Build history of the part. All positions in model axes, mm. A direction names the side the tool comes from. Round coordinates to 2 decimals unless told otherwise and drop trailing zeros. Order: outer loops, then holes, each group sorted by start corner. A loop starts at its lowest first (then second) coordinate and runs counter-clockwise, first axis right, second up. Notation, with made-up numbers: (61.5, 8) -> (113.5, 8) arc R23 ccw to (113.5, 28) -> close; hole circle Ø10 at (89.5, 67.5). An arc over 180 degrees is marked (long way). Answer as a JSON object with one key per item and string values.
from build123d import *

# Parameters (mm, degrees)
SKETCH_1_R          = 1.6
EXTRUDE_1_DEPTH     = 2
CUT_EXTRUDE_1_DEPTH = 88.4814266


with BuildPart() as part:
    # 草图1 → 凸台-拉伸1 (new body)
    with BuildSketch(Plane.XY):
        Polygon((0, 0), (0, 30), (25, 68), (55, 68), (55, 58), (44.157894737, 58), (6, 0), align=None)
        with Locations((3, 25)):
            Circle(SKETCH_1_R, mode=Mode.SUBTRACT)
        with Locations((3, 5)):
            Circle(SKETCH_1_R, mode=Mode.SUBTRACT)
        with Locations((30, 65)):
            Circle(SKETCH_1_R, mode=Mode.SUBTRACT)
        with Locations((50, 65)):
            Circle(SKETCH_1_R, mode=Mode.SUBTRACT)
    extrude(amount=EXTRUDE_1_DEPTH)

    # 草图2 → 切除-拉伸1 (cut, through all)
    with BuildSketch(Plane.XY.offset(2)):
        with BuildLine():
            Line((35.120951799, 58), (38.711972457, 58))
            ThreePointArc((38.711972457, 58), (39.592204387, 57.474543727), (39.547389539, 56.450383499))
            Line((39.547389539, 56.450383499), (29.621611135, 41.363200325))
            ThreePointArc((29.621611135, 41.363200325), (28.988285582, 40.933450188), (28.236577552, 41.077399744))
            Line((28.236577552, 41.077399744), (25.730326305, 42.726249249))
            ThreePointArc((25.730326305, 42.726249249), (25.300576167, 43.359574802), (25.444525724, 44.111282833))
            Line((25.444525724, 44.111282833), (34.285534717, 57.549616501))
            ThreePointArc((34.285534717, 57.549616501), (34.646408072, 57.88023193), (35.120951799, 58))
        make_face()
        with BuildLine():
            Line((8, 11.837801866), (8, 17.296153265))
            ThreePointArc((8, 17.296153265), (8.042028946, 17.583018145), (8.164582918, 17.845769767))
            Line((8.164582918, 17.845769767), (21.597210214, 38.263363257))
            ThreePointArc((21.597210214, 38.263363257), (22.230535767, 38.693113395), (22.982243798, 38.549163838))
            Line((22.982243798, 38.549163838), (25.488495044, 36.900314333))
            ThreePointArc((25.488495044, 36.900314333), (25.918245182, 36.26698878), (25.774295625, 35.51528075))
            Line((25.774295625, 35.51528075), (9.835417082, 11.288185364))
            ThreePointArc((9.835417082, 11.288185364), (8.713135121, 10.879830812), (8, 11.837801866))
        make_face()
    extrude(amount=-CUT_EXTRUDE_1_DEPTH, mode=Mode.SUBTRACT)


solid = part.part
1) Cut at A-A, the plane x = 50. Give the cut face in (y, z).
Checked values:
{"outline": "(58, 0) -> (63.4, 0) -> (63.4, 2) -> (58, 2) -> close; (66.6, 0) -> (68, 0) -> (68, 2) -> (66.6, 2) -> close"}
2) Which spindle directions (+Z, -Z, +X, -X, +Y, -Y) get a long thin tool onto all of the face, cutting with end or side? Do faces 5 (the face through (24, 42, 2)), 6 (the face through (14.787, 27.912, 1.014)). Say none if no direction does.
Checked values:
{"face 5": "+Z, +X, -X, +Y, -Y", "face 6": "+Z, -Z"}
3) Cut at B-B, the plane y = 52.5. Give the cut face in (x, z), plus the area to 3 significant figures.
Checked values:
{"outline": "(14.8, 0) -> (30.96, 0) -> (30.96, 2) -> (14.8, 2) -> close; (36.95, 0) -> (40.54, 0) -> (40.54, 2) -> (36.95, 2) -> close", "area": "39.5 mm²"}
4) Cut at D-D, the plane x = 30.5. Give the cut face in (y, z), plus the area to 3 significant figures.
Checked values:
{"outline": "(37.24, 0) -> (42.7, 0) -> (42.7, 2) -> (37.24, 2) -> close; (51.8, 0) -> (63.48, 0) -> (63.48, 2) -> (51.8, 2) -> close; (66.52, 0) -> (68, 0) -> (68, 2) -> (66.52, 2) -> close", "area": "37.2 mm²"}
5) Flat gauge pins, fed straight in: pin 1 Ø5 at (x, y) = (3, 5) entering from -Z; pin 2 Ø1 at (y, z) = (15, 1) entering from +X; pin 3 Ø1 at (x, z) = (51, 1) entering from -Y; pin 4 Ø12 at (x, y) = (38.5, 30.5) entering from +Z. Where does each tip first touch, or does it go through?
Checked values:
{"pin 1": "stops at z = 0", "pin 2": "stops at x = 16.2", "pin 3": "stops at y = 58", "pin 4": "passes through"}
6) Pull direction Y, two halves, no side cores. Call faces 1 (the face through (50, 58, 1)), 2 (the face through (55, 63, 1)), 3 (the face through (12.325, 48.734, 0.986)), 4 (the face through (39.585, 57.488, 1.014)): pulls with the +Y half, pulls with the -Y half, needs draft (parallel to the pull), parting line crosses it, or undercut.
Checked values:
{"face 1": "pulls with the -Y half", "face 2": "needs draft", "face 3": "pulls with the +Y half", "face 4": "undercut"}
7) Cut at C-C, the plane z = 0.75. Give the cut face in (x, y), plus the area to 3 significant figures.
Checked values:
{"outline": "(0, 0) -> (6, 0) -> (44.16, 58) -> (55, 58) -> (55, 68) -> (25, 68) -> (0, 30) -> close; hole circle Ø3.2 at (3, 5); hole circle Ø3.2 at (3, 25); hole (8, 11.84) arc R1 ccw to (9.84, 11.29) -> (25.77, 35.52) arc R1 ccw to (25.49, 36.9) -> (22.98, 38.55) arc R1 ccw to (21.6, 38.26) -> (8.16, 17.85) arc R1 ccw to (8, 17.3) -> close; hole (25.44, 44.11) arc R1 ccw to (25.73, 42.73) -> (28.24, 41.08) arc R1 ccw to (29.62, 41.36) -> (39.55, 56.45) arc R1 ccw to (38.71, 58) -> (35.12, 58) arc R1 ccw to (34.29, 57.55) -> close; hole circle Ø3.2 at (30, 65); hole circle Ø3.2 at (50, 65)", "area": "1,260 mm²"}
8) Probe L1, parallel to Y at x = 30, z = 1.55; L2, parallel to Y at x = 3, z = 1.15; L3, parallel to Y at x = 50, z = 1.6. List the from-to ranges inside material, lowest first. Write a range as from..to.
Checked values:
{"L1": "y = 36.48..41.94, 51.04..63.4, 66.6..68", "L2": "y = 0..3.4, 6.6..23.4, 26.6..34.56", "L3": "y = 58..63.4, 66.6..68"}
